Geometry check sheet. Reference: drawing and pictorial views, mm from the part's lowest x, y, z. A direction names the side the tool comes from. Round coordinates to 2 decimals unless told otherwise and drop trailing zeros. Loops run counter-clockwise (first coordinate to the right, second up) from the corner with the lowest first, then second, coordinate; pieces in that order, holes last. Notation, with made-up numbers: M 7,21.5 L 24,21.5 A6 cw 24,32.5 Z; hole C 51.25,6.5 d10. An arc over 180 degrees is marked long. One line per question, with ' | ' between items. Start each with the question number.
(1) Section check A-A (x = 2.05). Record the boundary of the cut face in (y, z).
(2) Section check D-D (x = 5.5). Record the boundary of the cut face in (y, z).
(3) Go/stop test with flat-tipped pins: P1, Ø2.5, axis at y = 21, z = 4.5, coming from the -X side; P2, Ø2.5, axis at x = 29.75, z = 6.25, coming from the -Y side; P3, Ø1, axis at x = 13.5, z = 1.5, coming from the +Y side. Record where each tip stops, or that it passes through.
(4) Thickness scan on probe 1 along Z at (x, y) = (2.05, 16.6); probe 2 along Y at (x, z) = (10, 9.75); probe 3 along Y at (x, z) = (4.5, 8.25). Record the ranges inside material, lowest first. Write a range as [from, to].
(5) Section check C-C (z = 3). Record the boundary of the cut face in (x, y).
(6) Tool access check on the marked faces 4, 5 and 6. Record the directions out of +Z, -Z, +X, -X, +Y, -Y that give a thin tool (end or side, any length) a straight path to the whole face; none if there is none.
(7) Draft check along Y on the marked faces 1, 2 and 3. Enter one of: +Y half, -Y half, draft (parallel to the pull), parting line (faces both ways), or undercut.
(8) Section check B-B (y = 17). Record the boundary of the cut face in (x, z).
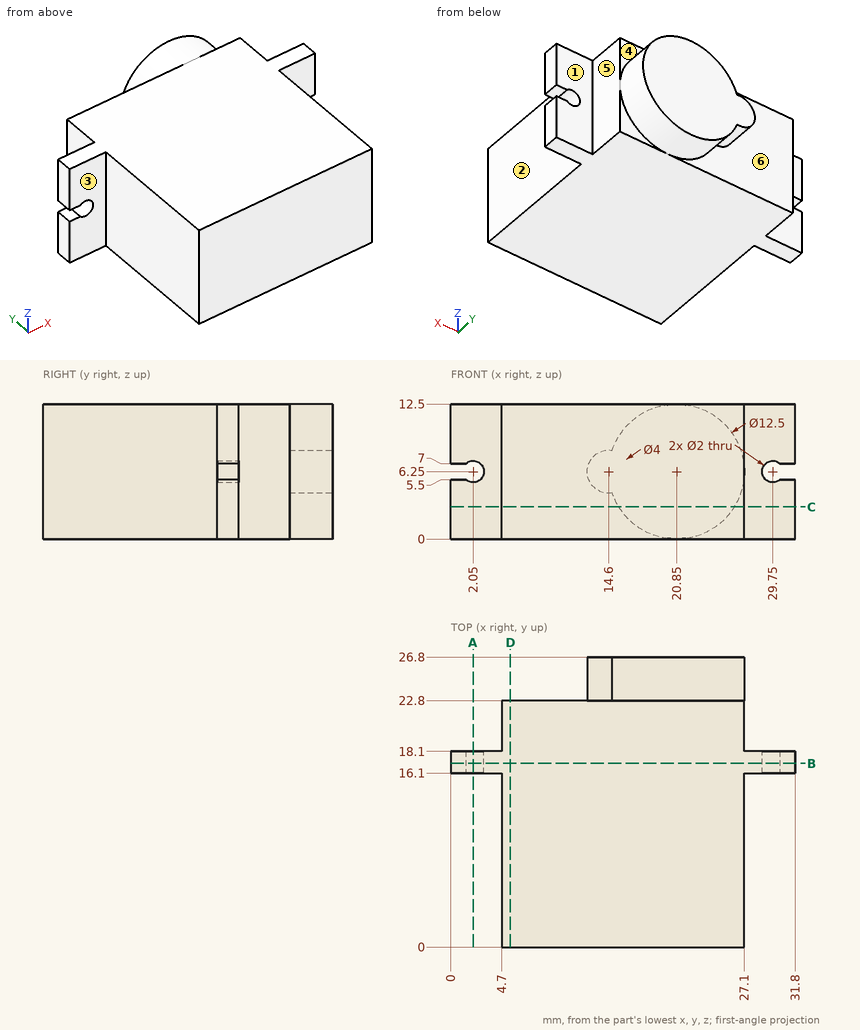
The answers:
1) outline: M 16.1,0 L 18.1,0 L 18.1,5.25 L 16.1,5.25 Z; M 16.1,7.25 L 18.1,7.25 L 18.1,12.5 L 16.1,12.5 Z
2) outline: M 0,0 L 22.8,0 L 22.8,12.5 L 0,12.5 Z
3) P1: x = 4.7 | P2: y = 16.1 | P3: y = 22.8
4) probe 1: [0, 5.25], [7.25, 12.5] | probe 2: [0, 22.8] | probe 3: [16.1, 18.1]
5) outline: M 0,16.1 L 4.7,16.1 L 4.7,0 L 27.1,0 L 27.1,16.1 L 31.8,16.1 L 31.8,18.1 L 27.1,18.1 L 27.1,22.8 L 26.19,22.8 L 26.19,26.8 L 15.51,26.8 L 15.51,22.8 L 4.7,22.8 L 4.7,18.1 L 0,18.1 Z
6) face 4: +Z, +X, +Y | face 5: +Z, -Z, +X, +Y | face 6: -X, +Y
7) face 1: +Y half | face 2: draft | face 3: -Y half
8) outline: M 0,0 L 31.8,0 L 31.8,5.5 L 30.41,5.5 A1 cw long 30.41,7 L 31.8,7 L 31.8,12.5 L 0,12.5 L 0,7 L 1.39,7 A1 cw long 1.39,5.5 L 0,5.5 Z
